Check sheet for the modelled part. Datum: model origin and axes. Units: mm. A direction names the side the tool comes from. Round coordinates to 2 decimals unless told otherwise and drop trailing zeros. Write each loop counter-clockwise with the first axis right and the second up, starting at its lowest first coordinate (ties: lowest second). Pieces come first, ordered by that corner, then holes. Notation, with made-up numbers: (10.25, 1.5) -> (17.25, 1.5) arc R27 ccw to (17.25, 26.5) -> close; hole circle Ø11 at (-24, 27). An arc over 180 degrees is marked (long way). One line per item, written item: value.
from build123d import *

# Parameters (mm, degrees)
F0_R     = 1.5875
F1_DEPTH = 3.048


with BuildPart() as f1:
    # F0 (on Front) → F1 (new body)
    with BuildSketch(Plane.XZ):
        with BuildLine():
            ThreePointArc((44.7324052746, -7.9324746146), (50.1616327839, -5.5119104847), (52.3875, 0))
            ThreePointArc((52.3875, 0), (50.0626600757, 5.6126600757), (44.45, 7.9375))
            ThreePointArc((44.45, 7.9375), (36.5137564458, -0.1412249921), (44.7324052746, -7.9324746146))
        make_face()
        with Locations((44.45, 0)):
            Circle(F0_R, mode=Mode.SUBTRACT)
        with BuildLine():
            ThreePointArc((44.7324052746, -7.9324746146), (36.5137564458, -0.1412249921), (44.45, 7.9375))
            Line((44.45, 7.9375), (18.8228170321, 8.8527565346))
            ThreePointArc((18.8228170321, 8.8527565346), (13.130598856, 11.5544736108), (11.1919966494, 17.549675393))
            Line((11.1919966494, 17.549675393), (15.0877196672, 58.5627598555))
            ThreePointArc((15.0877196672, 58.5627598555), (-0.0101583242, 47.6250032501), (-15.0940259351, 58.5820729906))
            Line((-15.0940259351, 58.5820729906), (-9.4828929283, -0.8946321652))
            ThreePointArc((-9.4828929283, -0.8946321652), (-0.4478112651, 9.5144674087), (9.525, 0))
            ThreePointArc((9.525, 0), (6.9705567315, -6.4912990883), (0.6773435479, -9.500885786))
            Line((0.6773435479, -9.500885786), (44.7324052746, -7.9324746146))
        make_face()
        with BuildLine():
            Line((0, -9.525), (0.6773435479, -9.500885786))
            ThreePointArc((0.6773435479, -9.500885786), (6.9705567315, -6.4912990883), (9.525, 0))
            ThreePointArc((9.525, 0), (-0.4478112651, 9.5144674087), (-9.4828929283, -0.8946321652))
            ThreePointArc((-9.4828929283, -0.8946321652), (-6.4110940418, -7.0443948063), (0, -9.525))
        make_face()
        Circle(F0_R, mode=Mode.SUBTRACT)
        with BuildLine():
            ThreePointArc((0, -9.525), (0.3388863295, -9.5189695375), (0.6773435479, -9.500885786))
            Line((0.6773435479, -9.500885786), (0, -9.525))
        make_face()
        with BuildLine():
            Line((15.7474569047, 65.5082893304), (15.0877196672, 58.5627598555))
            ThreePointArc((15.0877196672, 58.5627598555), (15.6769444522, 61.0001924791), (15.875, 63.5))
            ThreePointArc((15.875, 63.5), (15.8430821396, 64.5061676396), (15.7474569047, 65.5082893304))
        make_face()
        with BuildLine():
            ThreePointArc((-15.0940259351, 58.5820729906), (-0.0101583242, 47.6250032501), (15.0877196672, 58.5627598555))
            Line((15.0877196672, 58.5627598555), (15.7474569047, 65.5082893304))
            ThreePointArc((15.7474569047, 65.5082893304), (0, 79.375), (-15.7474569047, 65.5082893304))
            Line((-15.7474569047, 65.5082893304), (-15.0940259351, 58.5820729906))
        make_face()
        with Locations((0, 63.5)):
            Circle(F0_R, mode=Mode.SUBTRACT)
        with BuildLine():
            ThreePointArc((-15.7474569047, 65.5082893304), (-15.8048215471, 62.0089463914), (-15.0940259351, 58.5820729906))
            Line((-15.0940259351, 58.5820729906), (-15.7474569047, 65.5082893304))
        make_face()
        with BuildLine():
            ThreePointArc((-15.7474569047, 65.5082893304), (0, 79.375), (15.7474569047, 65.5082893304))
            Line((15.7474569047, 65.5082893304), (9.525, 114.3))
            ThreePointArc((9.525, 114.3), (0, 104.775), (-9.525, 114.3))
            Line((-9.525, 114.3), (-15.7474569047, 65.5082893304))
        make_face()
        with Locations((-1.5875, 101.5796237513)):
            Circle(F0_R, mode=Mode.SUBTRACT)
        with BuildLine():
            ThreePointArc((-9.525, 114.3), (0, 104.775), (9.525, 114.3))
            ThreePointArc((9.525, 114.3), (0, 123.825), (-9.525, 114.3))
        make_face()
        with Locations((0, 114.3)):
            Circle(F0_R, mode=Mode.SUBTRACT)
    extrude(amount=F1_DEPTH)


solid = f1.part
Item 1: Material ranges on line 1 along X through (y, z) = (-0.55, 114.3) (1 decimal); line 2 along X through (y, z) = (-1.45, 118); line 3 along Z through (x, y) = (34.5, -2.8), recorded low to high.
Result set:
line 1: -9.5 to -1.6, 1.6 to 9.5
line 2: -8.78 to 8.78
line 3: -8.3 to 8.29
Item 2: Release check for a two-part mould opening along Z. For faces 1 (the cylindrical face through (-0.34, -1.5, -1.55)), 2 (the cylindrical face through (0.209, -1.503, 123.823)), 3 (the cylindrical face through (52.387, -1.503, -0.031)) record: pulls with the +Z half, pulls with the -Z half, needs draft (parallel to the pull), parting line crosses it, or undercut.
Result set:
face 1: undercut
face 2: pulls with the +Z half
face 3: parting line crosses it
Item 3: Tool access check on faces 4 (the flat face through (13.113, -1.503, 37.769)), 5 (the flat face through (-12.328, -1.503, 29.26)). Record the directions out of +Z, -Z, +X, -X, +Y, -Y that give a thin tool (end or side, any length) a straight path to the whole face; none if there is none.
Result set:
face 4: +X, +Y, -Y
face 5: -Z, -X, +Y, -Y
Item 4: Sectioned sample at C-C (x = 40.5). Enter the section's corners in (y, z), then the cut area to 3 significant figures.
Result set:
outline: (-3.05, -8.08) -> (0, -8.08) -> (0, 8.08) -> (-3.05, 8.08) -> close
area: 49.3 mm^2
Item 5: Sectioned sample at B-B (z = 34). Enter the section's corners in (x, y), then the cut area to 3 significant figures.
Result set:
outline: (-12.77, -3.05) -> (12.75, -3.05) -> (12.75, 0) -> (-12.77, 0) -> close
area: 77.8 mm^2
Item 6: Depth check by flat-ended pin: pin 1 (4 mm diameter, centred on x = 10.5, z = 10, fed in from +Y); pin 2 (3 mm diameter, centred on x = -1.59, z = 101.58, fed in from +Y). Enter the tip coordinate at first touch or a pass-through.
Result set:
pin 1: y = 0
pin 2: through
Item 7: Sectioned sample at A-A (y = -1.15). State how many separate pieces and enclosed holes the cut face has, then the cut area to 3 significant figures.
Result set:
separate pieces: 1
enclosed holes: 5
area: 3,870 mm^2
